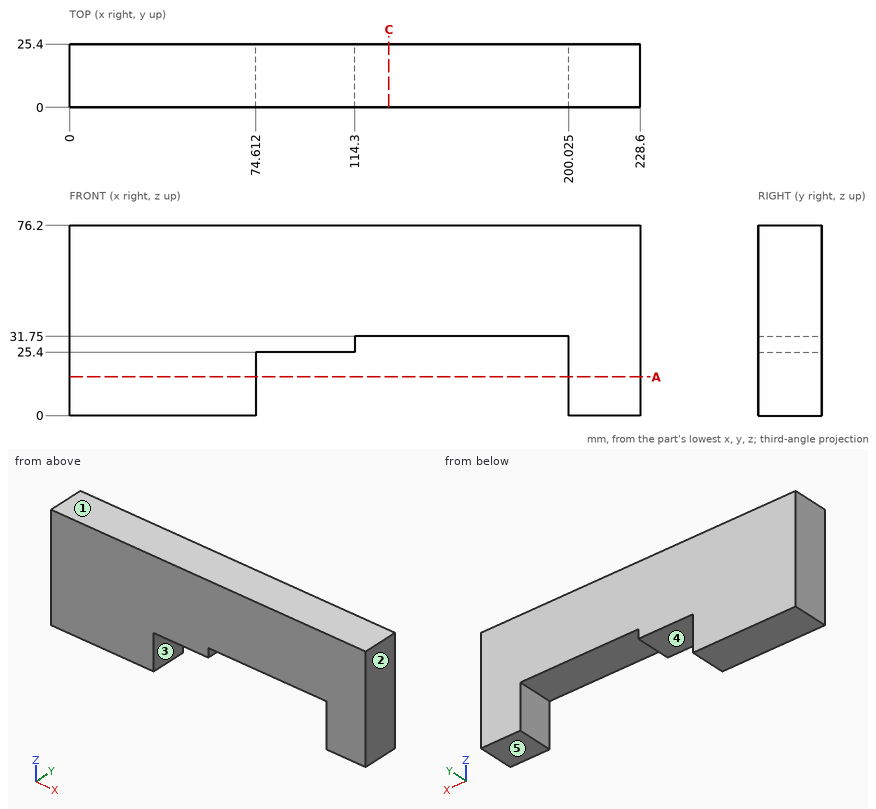
Job drawing, mm, ordinate dimensions from the low corner. One solid piece. A direction names the side the tool comes from. Coordinates: 2 decimals unless noted, no trailing zeros. Order: outer loops, then holes, each group sorted by start corner. A loop starts at its lowest first (then second) coordinate and runs counter-clockwise, first axis right, second up. Notation, with made-up numbers: (-16.75, 59.25) -> (35.25, 59.25) arc R12 cw to (35.25, 75.25) -> close; hole circle Ø8 at (-35, 1.25). An arc over 180 degrees is marked (long way). Put each result on its own line as item: value. Start each with the question number.
(1) Band-saw the part on A-A (z = 15.5). Give the cut face in (x, y) (1 decimal), then the cut area to 3 significant figures.
(2) Mould opens along X. For the marked faces 1, 2 and 3 say: pulls with the +X half, pulls with the -X half, needs draft (parallel to the pull), parting line crosses it, or undercut.
(3) Pin check, flat tips, straight feed: pin 1 Ø10 at (x, y) = (172, 3.5) entering from -Z; pin 2 Ø10 at (x, z) = (80, 10) entering from +Y; pin 3 Ø4 at (x, y) = (79.5, 18.5) entering from -Z. Stop position of each tip, or through.
(4) Which spindle directions (+Z, -Z, +X, -X, +Y, -Y) get a long thin tool onto all of the face, cutting with end or side? Do the marked faces 4 and 5. Say none if no direction does.
(5) Probe line 1 along X through (y, z) = (22.25, 18) (1 decimal); line 2 along Z through (x, y) = (169.5, 3.75); line 3 along X through (y, z) = (14.25, 26) (1 decimal). List the from-to ranges inside material, lowest first. Write a range as [from, to].
(6) Band-saw the part on C-C (x = 128). Give the cut face in (y, z).
Determined:
1. outline: (0, 0) -> (74.6, 0) -> (74.6, 25.4) -> (0, 25.4) -> close; (200, 0) -> (228.6, 0) -> (228.6, 25.4) -> (200, 25.4) -> close
1. area: 2,620 mm²
2. face 1: needs draft
2. face 2: pulls with the +X half
2. face 3: undercut
3. pin 1: stops at z = 31.75
3. pin 2: passes through
3. pin 3: stops at z = 25.4
4. face 4: -Z, +Y, -Y
4. face 5: -Z, +X, -X, +Y, -Y
5. line 1: x = [0, 74.6], [200, 228.6]
5. line 2: z = [31.75, 76.2]
5. line 3: x = [0, 114.3], [200, 228.6]
6. outline: (0, 31.75) -> (25.4, 31.75) -> (25.4, 76.2) -> (0, 76.2) -> close
